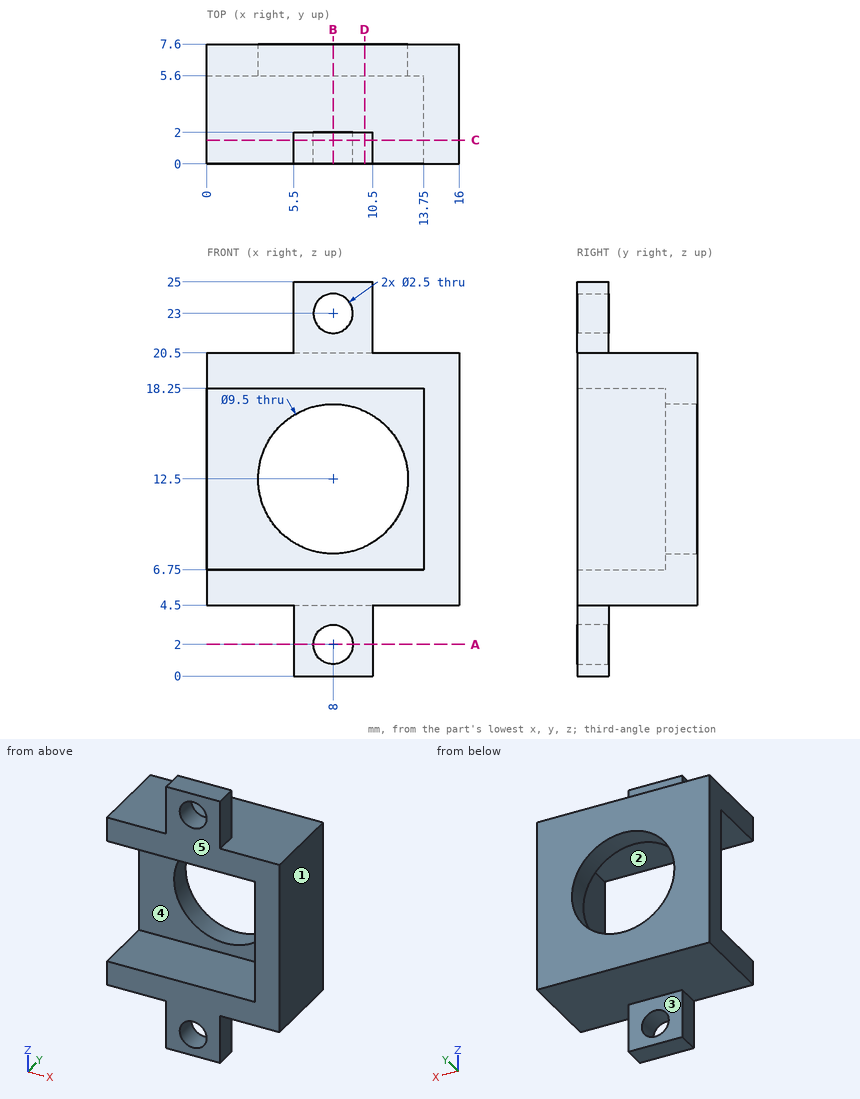
The drawing under review shows one solid part. Ordinate dimensions are in mm from its lowest x, y, z. A direction names the side the tool comes from. Coordinates: 2 decimals unless noted, no trailing zeros. Loops run counter-clockwise (first coordinate to the right, second up) from the corner with the lowest first, then second, coordinate; pieces in that order, holes last. Notation, with made-up numbers: (82.5, -22) - (102.5, -22) arc R21 ccw to (102.5, -4) - close; hole circle Ø1 at (-2, -36). An arc over 180 degrees is marked (long way). Use CSV: the item, a comma, the result in double quotes. Start each with the question number.
1. Add section C-C on y = 1.5. Give the boundary of the cut face in (x, z).
2. Mouldability with a two-part tool opening along Z and no side actions: class the marked faces 4 and 5 as released by +Z, released by -Z, zero draft, split by the parting line, or undercut.
3. For the marked faces 1, 2 and 3, list the 3-axis set-ups (+Z, -Z, +X, -X, +Y, -Y) from which the entire face can be reached by the end or side of a thin tool; tool diameter is ignored.
4. Add section B-B on x = 8. Give the boundary of the cut face in (y, z).
5. Add section A-A on z = 2. Give the boundary of the cut face in (x, y).
6. Clearance check with flat-ended pins moving along their axes: pin 1 (1.6 mm diameter, centred on y = 1.5, z = 2.5, fed in from +X); pin 2 (1.7 mm diameter, centred on y = 2.5, z = 13.5, fed in from -X); pin 3 (1.6 mm diameter, centred on y = 1.5, z = 3, fed in from -X); pin 4 (2 mm diameter, centred on x = 8, z = 23, fed in from -Y). State where each tip first meets the part, or that it passes through.
7. Add section D-D on x = 10. Give the boundary of the cut face in (y, z).
8. To check wall thickness, follow probe 1 along X at (y, z) = (1.2, 2); probe 2 along Z at (x, y) = (2, 1.5); probe 3 along X at (y, z) = (5, 7.25). State the ranges of each line that lie inside material, in increasing order.
Resolved:
1,outline,"(0, 4.5) - (5.5, 4.5) - (5.5, 0) - (10.5, 0) - (10.5, 4.5) - (16, 4.5) - (16, 20.5) - (10.5, 20.5) - (10.5, 25) - (5.5, 25) - (5.5, 20.5) - (0, 20.5) - (0, 18.25) - (13.75, 18.25) - (13.75, 6.75) - (0, 6.75) - close; hole circle Ø2.5 at (8, 2); hole circle Ø2.5 at (8, 23)"
2,face 4,"undercut"
2,face 5,"zero draft"
3,face 1,"+Z, -Z, +X, +Y, -Y"
3,face 2,"-X, -Y"
3,face 3,"-Z, +X, -X, +Y"
4,outline,"(0, 0) - (2, 0) - (2, 0.75) - (0, 0.75) - close; (0, 3.25) - (2, 3.25) - (2, 4.5) - (7.6, 4.5) - (7.6, 7.75) - (5.6, 7.75) - (5.6, 6.75) - (0, 6.75) - close; (0, 18.25) - (5.6, 18.25) - (5.6, 17.25) - (7.6, 17.25) - (7.6, 20.5) - (2, 20.5) - (2, 21.75) - (0, 21.75) - close; (0, 24.25) - (2, 24.25) - (2, 25) - (0, 25) - close"
5,outline,"(5.5, 0) - (6.75, 0) - (6.75, 2) - (5.5, 2) - close; (9.25, 0) - (10.5, 0) - (10.5, 2) - (9.25, 2) - close"
6,pin 1,"x = 10.5"
6,pin 2,"x = 13.75"
6,pin 3,"x = 5.5"
6,pin 4,"through"
7,outline,"(0, 0) - (2, 0) - (2, 4.5) - (7.6, 4.5) - (7.6, 8.19) - (5.6, 8.19) - (5.6, 6.75) - (0, 6.75) - close; (0, 18.25) - (5.6, 18.25) - (5.6, 16.81) - (7.6, 16.81) - (7.6, 20.5) - (2, 20.5) - (2, 25) - (0, 25) - close"
8,probe 1,"5.5 to 6.75, 9.25 to 10.5"
8,probe 2,"4.5 to 6.75, 18.25 to 20.5"
8,probe 3,"13.75 to 16"
